Geometry check sheet. Reference: the model listing, model coordinates, mm. Coordinates: 2 decimals unless noted, no trailing zeros.
from build123d import *

# Parameters (mm, degrees)
BOSS_EXTRUDE1_DEPTH             = 6.35
BOSS_EXTRUDE2_DEPTH             = 6.35
F_1_4_0_25_DIAMETER_HOLE2_D     = 6.35
F_1_4_0_25_DIAMETER_HOLE3_D     = 6.35
F_1_4_0_25_DIAMETER_HOLE3_DEPTH = 6.35


with BuildPart() as part:
    # Sketch1 → Boss-Extrude1 (new body)
    with BuildSketch(Plane.XY):
        with BuildLine():
            Line((0, 0), (739.14, 0))
            add(Edge.make_bspline(
                [(277.420636668, 567.826315519), (496.859161811, 420.297110317), (620.758181585, 229.590161119), (739.14, 0)],
                knots=[0, 0, 0, 0, 1, 1, 1, 1], degree=3))
            Line((277.420636668, 567.826315519), (64.695636668, 567.826315519))
            Line((64.695636668, 567.826315519), (0, 0))
        make_face()
    extrude(amount=BOSS_EXTRUDE1_DEPTH)

    # Sketch5 → Boss-Extrude2 (add)
    with BuildSketch(Plane(origin=(0, 0, 0), x_dir=(-1, 0, 0), z_dir=(0, 0, -1))):
        Polygon((-64.695636668, 567.826315519), (-32.740222655, 567.826315519), (31.955414013, 0), (0, 0), align=None)
    extrude(amount=-BOSS_EXTRUDE2_DEPTH)

    # 1/4 (0.25) Diameter Hole2 (through all)
    with Locations(Plane.XY.offset(6.35)):
        with Locations((-6.712513837, 75.710175403), (-0.961790578, 126.183625671), (39.293272238, 479.49777755), (45.043995497, 529.971227818)):
            Hole(F_1_4_0_25_DIAMETER_HOLE2_D / 2)

    # 1/4 (0.25) Diameter Hole3
    with Locations(Plane.XY.offset(6.35)):
        with Locations((720.09, 12.7), (267.895636668, 555.126315519)):
            Hole(F_1_4_0_25_DIAMETER_HOLE3_D / 2, depth=F_1_4_0_25_DIAMETER_HOLE3_DEPTH)


solid = part.part
1. Draft check along X on faces 1 (the flat face through (263, 225, 6.35)), 2 (the flat face through (0.845, 287.888, 3.131)). Enter one of: released by +X, released by -X, zero draft, split by the parting line, or undercut.
Computed values:
face 1: zero draft
face 2: released by -X
2. Gauge pin test, flat end, axial feed: pin 1 Ø2 at (x, z) = (475, 5.5) entering from +Y. Record the tip position at first contact, or that the pin passes through.
Computed values:
pin 1: stops at y = 400.02
3. Sectioned sample at A-A, the plane z = 2.5. Give the number of separate pieces and of enclosed holes in the cut face, and give its area (3 significant figures).
Computed values:
separate pieces: 1
enclosed holes: 6
area: 312,000 mm2
4. Thickness scan on line 1 along X through (y, z) = (346, 4.5); line 2 along X through (y, z) = (165, 2.25); line 3 along Y through (x, z) = (616.5, 3.5). Record the ranges inside material, lowest first.
Computed values:
line 1: x = 7.47 to 521.22
line 2: x = -13.16 to 647.81
line 3: y = 0 to 215.06
